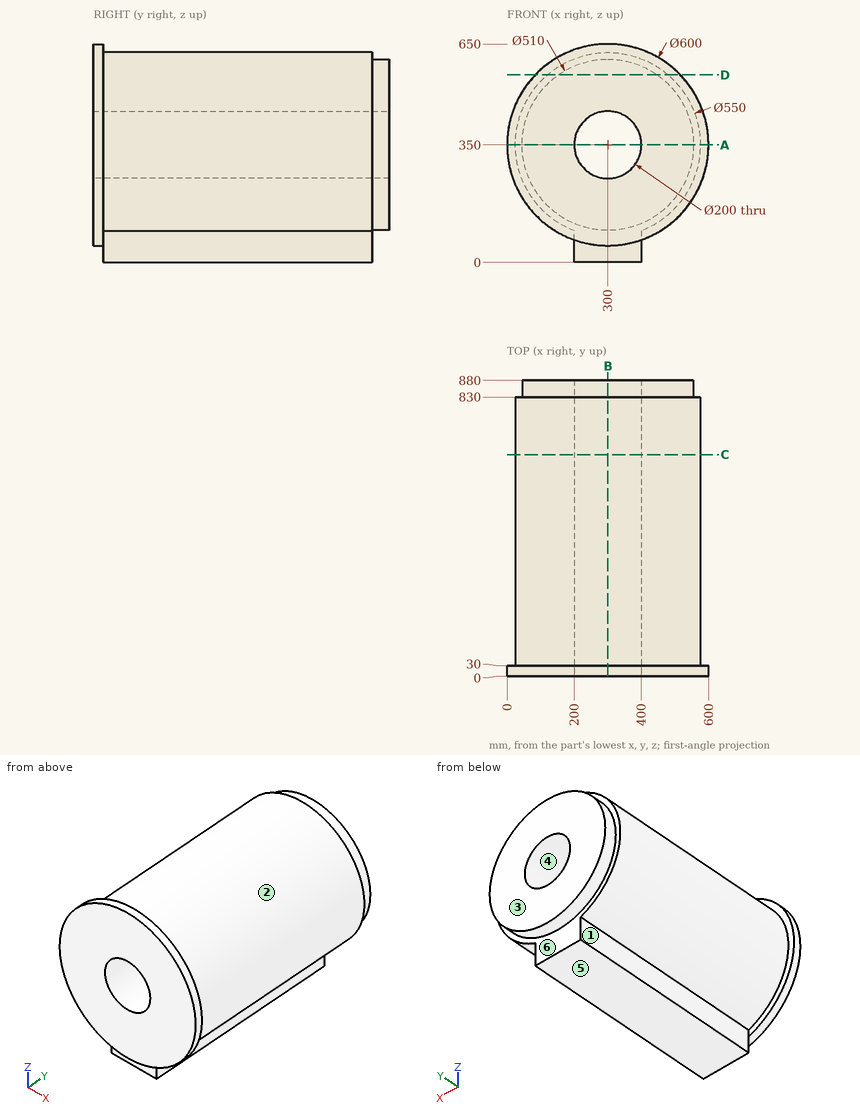
Print and shaded views of the part. All mm, measured from the part's lowest x, y and z. A direction names the side the tool comes from. Give positions to 0.01 mm unless a question says otherwise; leave off trailing zeros. Loops run counter-clockwise (first coordinate to the right, second up) from the corner with the lowest first, then second, coordinate; pieces in that order, holes last. Notation, with made-up numbers: M 76,31.5 L 99,31.5 A25 ccw 99,55.5 Z; hole C 43,82.25 d1. An arc over 180 degrees is marked long. Write each question's results on one line, items separated by ' | '.
Q1. Band-saw the part on D-D on z = 558. Write the cut outline in (x, y), and give its area (3 significant figures).
Geometry check:
outline: M 83.81,0 L 516.19,0 L 516.19,30 L 479.89,30 L 479.89,830 L 447.52,830 L 447.52,880 L 152.48,880 L 152.48,830 L 120.11,830 L 120.11,30 L 83.81,30 Z | area: 316,000 mm²
Q2. Mould opens along Z. For the marked faces 4, 5 and 6 say: pulls with the +Z half, pulls with the -Z half, needs draft (parallel to the pull), parting line crosses it, or undercut.
Geometry check:
face 4: undercut | face 5: pulls with the -Z half | face 6: needs draft
Q3. Band-saw the part on C-C on y = 659. Write the cut outline in (x, z), and give its area (3 significant figures).
Geometry check:
outline: M 200,0 L 400,0 L 400,93.83 A275 ccw long 200,93.83 Z; hole C 300,350 d200 | area: 222,000 mm²
Q4. Flat gauge pins, fed straight in: P1, Ø4, axis at x = 161.5, y = 511.5, coming from the +Z side; P2, Ø5, axis at y = 446.5, z = 279.5, coming from the -X side; P3, Ø12, axis at x = 220.5, z = 395, coming from the +Y side; P4, Ø2, axis at x = 416.5, y = 100, coming from the +Z side. Where does each tip first touch, or does it go through?
Geometry check:
P1: stops at z = 588.73 | P2: stops at x = 33.54 | P3: passes through | P4: stops at z = 599.57
Q5. Probe probe 1 along X at (y, z) = (547, 350); probe 2 along Y at (x, z) = (234, 601); probe 3 along Z at (x, y) = (225, 528.5). List the from-to ranges inside material, lowest first.
Geometry check:
probe 1: x = 25 to 200, 400 to 575 | probe 2: y = 0 to 830 | probe 3: z = 0 to 283.86, 416.14 to 614.58
Q6. Band-saw the part on B-B on x = 300. Write the cut outline in (y, z), and give its area (4 significant figures).
Geometry check:
outline: M 0,50 L 30,50 L 30,0 L 830,0 L 830,95 L 880,95 L 880,250 L 0,250 Z; M 0,450 L 880,450 L 880,605 L 830,605 L 830,625 L 30,625 L 30,650 L 0,650 Z | area: 367,500 mm²
Q7. Band-saw the part on A-A on z = 350. Write the cut outline in (x, y), and give its area (4 significant figures).
Geometry check:
outline: M 0,0 L 200,0 L 200,880 L 45,880 L 45,830 L 25,830 L 25,30 L 0,30 Z; M 400,0 L 600,0 L 600,30 L 575,30 L 575,830 L 555,830 L 555,880 L 400,880 Z | area: 307,500 mm²
Q8. Which spindle directions (+Z, -Z, +X, -X, +Y, -Y) get a long thin tool onto all of the face, cutting with end or side? Do the marked faces 1, 2 and 3. Say none if no direction does.
Geometry check:
face 1: -Z, -X, +Y | face 2: +Y | face 3: +Z, -Z, +X, -X, +Y
